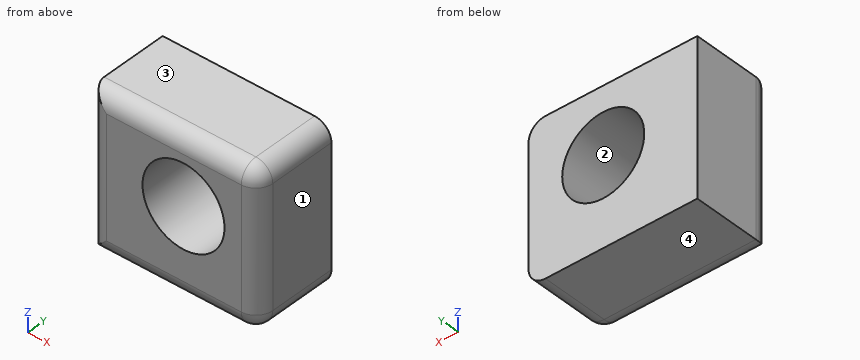
```python
from build123d import *

# Parameters (mm, degrees)
F0_W     = 50.8
F0_H     = 25.4
F1_DEPTH = 46.482
F2_R     = 12.351013
F3_DEPTH = 25.4
F4_R     = 5.08
F5_R     = 5.08


with BuildPart() as f1:
    # F0 (on Top) → F1 (new body)
    with BuildSketch(Plane.XY):
        with Locations((25.4, 12.7)):
            Rectangle(F0_W, F0_H)
    extrude(amount=F1_DEPTH)

    # F2 (on face) → F3 (cut)
    with BuildSketch(Plane.XZ):
        with Locations((28.329594, 26.583312)):
            Circle(F2_R)
    extrude(amount=-F3_DEPTH, mode=Mode.SUBTRACT)

    # F4
    f4_edges = [f1.edges().sort_by_distance(p)[0] for p in [
        (50.8, 0, 23.241),
    ]]
    fillet(f4_edges, radius=F4_R)

    # F5
    f5_edges = [f1.edges().sort_by_distance(p)[0] for p in [
        (22.86, 0, 0),
        (0, 0, 23.241),
        (22.86, 0, 46.482),
    ]]
    fillet(f5_edges, radius=F5_R)


solid = f1.part
```
Part model, mm, in its own coordinate system. Face numbers are marked on the shaded views. Give positions to 0.01 mm unless a question says otherwise; leave off trailing zeros. Order: outer loops, then holes, each group sorted by start corner. A loop starts at its lowest first (then second) coordinate and runs counter-clockwise, first axis right, second up. Notation, with made-up numbers: M -6.5,35.5 L 26.5,35.5 A9 cw 26.5,44.5 Z; hole C 51,88 d9. An arc over 180 degrees is marked long. Use a Markdown table: item, result. Add a question column.
(1) Saw through at B-B, the plane z = 28. Give the cut face in (x, y), and give its area (3 significant figures).
(2) Mould opens along Z. For the marked faces 1, 2, 3 and 4 say: +Z half, -Z half, draft (parallel to the pull), parting line (faces both ways), or undercut.
(3) Saw through at A-A, the plane x = 32. Give the cut face in (y, z), and give its area (3 significant figures).
(4) Saw through at C-C, the plane y = 7.5. Give the cut face in (x, z), and give its area (3 significant figures).
(5) Saw through at D-D, the plane z = 43. Give the cut face in (x, y), and give its area (3 significant figures).
(6) Probe line 1 along X through (y, z) = (21, 26); line 2 along X through (y, z) = (4.75, 40.5); line 3 along Z through (x, y) = (34.5, 19). List the from-to ranges inside material, lowest first. Write a range as [from, to].
Answer key:
| question | item | result |
|---|---|---|
| 1 | outline | M 0,5.08 A5.08 ccw 5.08,0 L 16.06,0 L 16.06,25.4 L 0,25.4 Z; M 40.6,0 L 45.72,0 A5.08 ccw 50.8,5.08 L 50.8,25.4 L 40.6,25.4 Z |
| 1 | area | 656 mm^2 |
| 2 | face 1 | draft |
| 2 | face 2 | undercut |
| 2 | face 3 | +Z half |
| 2 | face 4 | -Z half |
| 3 | outline | M 0,5.08 A5.08 ccw 5.08,0 L 25.4,0 L 25.4,14.79 L 0,14.79 Z; M 0,38.38 L 25.4,38.38 L 25.4,46.48 L 5.08,46.48 A5.08 ccw 0,41.4 Z |
| 3 | area | 570 mm^2 |
| 4 | outline | M 0,0 L 45.72,0 A5.08 ccw 50.8,5.08 L 50.8,41.4 A5.08 ccw 45.72,46.48 L 0,46.48 Z; hole C 28.33,26.58 d24.7 |
| 4 | area | 1,870 mm^2 |
| 5 | outline | M 0,5.08 A5.08 ccw 3.48,0.26 L 45.72,0.26 A4.82 ccw 50.54,5.08 L 50.54,25.4 L 0,25.4 Z |
| 5 | area | 1,260 mm^2 |
| 6 | line 1 | [0, 15.99], [40.67, 50.8] |
| 6 | line 2 | [0.01, 50.79] |
| 6 | line 3 | [0, 15.88], [37.28, 46.48] |
